Source: CAD feature listing. Evaluate the final solid. Frame: model axes, mm. A direction names the side the tool comes from. Round coordinates to 2 decimals unless told otherwise and drop trailing zeros. Loops run counter-clockwise (first coordinate to the right, second up) from the corner with the lowest first, then second, coordinate; pieces in that order, holes last. Notation, with made-up numbers: M 19,-5.5 L 51,-5.5 A33 ccw 51,27.5 Z; hole C 3.25,48 d7. An arc over 180 degrees is marked long. Write each question's results on one line, items separated by ' | '. Start each with the question number.
1. Ray query, line 1 (Z direction, x = -12, y = 0.7); line 2 (Z direction, x = 7, y = -2.75) (3 decimals); line 3 (Z direction, x = -16.5, y = -2.3) (3 decimals). Return the intervals inside material, ascending.
2. Set-up query: faces 3 (the flat face through (20, 1.85, -4)), 4 (the cylindrical face through (-4.813, -2.24, -0.702)), 5 (the flat face through (0, 0, 0)). Return all of +Z, -Z, +X, -X, +Y, -Y with unobstructed straight access to the full face (end or side cutting, diameter ignored); none if empty.
3. Section A-A on z = 7.25. Output: boundary loops of the cut face in (x, y) (3 decimals).
4. Draft query along X for faces 1 (the flat face through (12, 1.85, -4)), 2 (the cylindrical face through (-4.35, -0.59, -3.08)). Return one class per face: released by +X, released by -X, zero draft, split by the parting line, or undercut.
5. Contact query for flat-ended pins moving along their axis: pin 1 Ø2.5 at (x, z) = (-8, -0.5) entering from -Y; pin 2 Ø5.5 at (x, z) = (-24, 1) entering from -Y; pin 3 Ø1 at (x, z) = (12, -4) entering from -Y. Output: stop coordinate, or through.
from build123d import *

# Parameters (mm, degrees)
SKETCH1_W           = 63.83
SKETCH1_H           = 15.83
BOSS_EXTRUDE1_DEPTH = 3.2
SKETCH2_R           = 2.45
BOSS_EXTRUDE2_DEPTH = 1.85
SHELL1_T            = -1.5
SKETCH3_R           = 3.24
SKETCH3_R_2         = 2.43
BOSS_EXTRUDE3_DEPTH = 1.5


with BuildPart() as part:
    # Sketch1 → Boss-Extrude1 (new body)
    with BuildSketch(Plane(origin=(0, 0, 0), x_dir=(1, 0, 0), z_dir=(0, 1, 0))):
        Rectangle(SKETCH1_W, SKETCH1_H)
    extrude(amount=-BOSS_EXTRUDE1_DEPTH)

    # Sketch2 → Boss-Extrude2 (add)
    with BuildSketch(Plane(origin=(0, 0, 0), x_dir=(1, 0, 0), z_dir=(0, 1, 0))):
        with Locations(Location((-27.925625, 3.9575, 0), (0, 0, 270))):
            Circle(SKETCH2_R)
        with Locations(Location((-19.945625, 3.9575, 0), (0, 0, 270))):
            Circle(SKETCH2_R)
        with Locations(Location((-11.965625, 3.9575, 0), (0, 0, 270))):
            Circle(SKETCH2_R)
        with Locations(Location((-3.985625, 3.9575, 0), (0, 0, 270))):
            Circle(SKETCH2_R)
        with Locations(Location((3.994375, 3.9575, 0), (0, 0, 270))):
            Circle(SKETCH2_R)
        with Locations(Location((11.974375, 3.9575, 0), (0, 0, 270))):
            Circle(SKETCH2_R)
        with Locations(Location((19.954375, 3.9575, 0), (0, 0, 270))):
            Circle(SKETCH2_R)
        with Locations(Location((27.934375, 3.9575, 0), (0, 0, 270))):
            Circle(SKETCH2_R)
        with Locations(Location((27.934375, -3.9575, 0), (0, 0, 90))):
            Circle(SKETCH2_R)
        with Locations(Location((19.954375, -3.9575, 0), (0, 0, 90))):
            Circle(SKETCH2_R)
        with Locations(Location((11.974375, -3.9575, 0), (0, 0, 90))):
            Circle(SKETCH2_R)
        with Locations(Location((3.994375, -3.9575, 0), (0, 0, 90))):
            Circle(SKETCH2_R)
        with Locations(Location((-3.985625, -3.9575, 0), (0, 0, 90))):
            Circle(SKETCH2_R)
        with Locations(Location((-11.965625, -3.9575, 0), (0, 0, 90))):
            Circle(SKETCH2_R)
        with Locations(Location((-19.945625, -3.9575, 0), (0, 0, 90))):
            Circle(SKETCH2_R)
        with Locations(Location((-27.925625, -3.9575, 0), (0, 0, 90))):
            Circle(SKETCH2_R)
    extrude(amount=BOSS_EXTRUDE2_DEPTH)

    # Shell1
    shell1_openings = [part.faces().sort_by_distance(p)[0] for p in [
        (0, -3.2, 0),
    ]]
    offset(amount=SHELL1_T, openings=shell1_openings, kind=Kind.INTERSECTION)

    # Sketch3 → Boss-Extrude3 (add)
    # profile 1 of 7: a face of its own
    with BuildSketch(Plane.XZ.offset(1.5)):
        with Locations(Location((-23.93625, 0, 0), (0, 0, 90))):
            Circle(SKETCH3_R)
        with Locations(Location((-23.93625, 0, 0), (0, 0, 90))):
            Circle(SKETCH3_R_2, mode=Mode.SUBTRACT)
    # profile 2 of 7: a face of its own
    with BuildSketch(Plane.XZ.offset(1.5)):
        with Locations(Location((-15.95625, 0, 0), (0, 0, 90))):
            Circle(SKETCH3_R)
        with Locations(Location((-15.95625, 0, 0), (0, 0, 90))):
            Circle(SKETCH3_R_2, mode=Mode.SUBTRACT)
    # profile 3 of 7: a face of its own
    with BuildSketch(Plane.XZ.offset(1.5)):
        with Locations(Location((-7.97625, 0, 0), (0, 0, 90))):
            Circle(SKETCH3_R)
        with Locations(Location((-7.97625, 0, 0), (0, 0, 90))):
            Circle(SKETCH3_R_2, mode=Mode.SUBTRACT)
    # profile 4 of 7: a face of its own
    with BuildSketch(Plane.XZ.offset(1.5)):
        with Locations(Location((0.00375, 0, 0), (0, 0, 90))):
            Circle(SKETCH3_R)
        with Locations(Location((0.00375, 0, 0), (0, 0, 90))):
            Circle(SKETCH3_R_2, mode=Mode.SUBTRACT)
    # profile 5 of 7: a face of its own
    with BuildSketch(Plane.XZ.offset(1.5)):
        with Locations(Location((7.98375, 0, 0), (0, 0, 90))):
            Circle(SKETCH3_R)
        with Locations(Location((7.98375, 0, 0), (0, 0, 90))):
            Circle(SKETCH3_R_2, mode=Mode.SUBTRACT)
    # profile 6 of 7: a face of its own
    with BuildSketch(Plane.XZ.offset(1.5)):
        with Locations(Location((15.96375, 0, 0), (0, 0, 90))):
            Circle(SKETCH3_R)
        with Locations(Location((15.96375, 0, 0), (0, 0, 90))):
            Circle(SKETCH3_R_2, mode=Mode.SUBTRACT)
    # profile 7 of 7: a face of its own
    with BuildSketch(Plane.XZ.offset(1.5)):
        with Locations(Location((23.94375, 0, 0), (0, 0, 90))):
            Circle(SKETCH3_R)
        with Locations(Location((23.94375, 0, 0), (0, 0, 90))):
            Circle(SKETCH3_R_2, mode=Mode.SUBTRACT)
    extrude(amount=BOSS_EXTRUDE3_DEPTH)


solid = part.part
Taken from the geometry:
1) line 1: -6.41 to -1.51, 1.51 to 6.41 | line 2: -7.915 to -6.415, -3.087 to -2.222, 2.222 to 3.087, 6.415 to 7.915 | line 3: -7.915 to -6.415, -3.194 to -2.368, 2.368 to 3.194, 6.415 to 7.915
2) face 3: +Z, -Z, +X, -X, +Y | face 4: -Y | face 5: +Y
3) outline: M -31.915,-3.2 L 31.915,-3.2 L 31.915,0 L -31.915,0 Z
4) face 1: zero draft | face 2: undercut
5) pin 1: y = -1.5 | pin 2: y = -3 | pin 3: y = 0.35
